Autodesk Inventor part; units mm, degrees
ref_plane "Work Plane1" through (29, -114.6, 0) normal (0, -1, 0) x (1, 0, 0)
ref_plane "YZ Plane" through (0, 0, 0) normal (1, 0, 0) x (0, 1, 0)
ref_plane "XZ Plane" through (0, 0, 0) normal (0, 1, 0) x (-1, 0, 0)
sketch "Sketch1" plane through (0, 0, 0) normal (0, 0, 1) x (1, 0, 0)
  line L0 (29, -258.2) -> (29, -233.2)
  line L1 (29, -233.2) -> (25, -233.2)
  line L2 (25, -233.2) -> (25, -193.2)
  line L3 (25, -193.2) -> (29, -193.2)
  line L4 (29, -193.2) -> (29, -168.2)
  line L5 (29, -168.2) -> (25, -168.2)
  line L6 (25, -168.2) -> (25, -128.2)
  line L7 (25, -128.2) -> (29, -128.2)
  line L8 (29, -128.2) -> (29, -103.2)
  line L9 (29, -103.2) -> (25, -103.2)
  line L10 (25, -103.2) -> (25, -63.2)
  line L11 (25, -63.2) -> (29, -63.2)
  line L12 (29, -63.2) -> (29, -36)
  line L13 (29, -36) -> (25, -36)
  line L14 (25, -36) -> (25, 4)
  line L15 (25, 4) -> (29, 4)
  line L16 (29, 4) -> (29, 29)
  line L17 (29, 29) -> (29, 25)
  line L18 (29, 25) -> (69, 25)
  line L19 (29, -258.2) -> (29, -254.2)
  line L20 (29, -254.2) -> (69, -254.2)
  line L21 (49, 25) -> (49, 50.1757)
  line L22 (69, -63.2) -> (69, -36)
  line L23 (73, -36) -> (73, 4)
  line L24 (69, -36) -> (73, -36)
  line L25 (73, 4) -> (69, 4)
  line L26 (73, -233.2) -> (73, -193.2)
  line L27 (73, -193.2) -> (69, -193.2)
  line L28 (69, -233.2) -> (73, -233.2)
  line L29 (69, -168.2) -> (73, -168.2)
  line L30 (73, -168.2) -> (73, -128.2)
  line L31 (73, -63.2) -> (69, -63.2)
  line L32 (69, -103.2) -> (73, -103.2)
  line L33 (73, -128.2) -> (69, -128.2)
  line L34 (73, -103.2) -> (73, -63.2)
  line L35 (69, 25) -> (69, 4)
  line L36 (69, -36) -> (69, -63.2)
  line L37 (69, -103.2) -> (69, -128.2)
  line L38 (69, -168.2) -> (69, -193.2)
  line L39 (69, -233.2) -> (69, -254.2)
  point P0 (0, 0)
  dimension "d1" = 40
  dimension "d2" = 4
  dimension "d3" = 40
  dimension "d4" = 40
  dimension "d5" = 40
  dimension "d6" = 40
  dimension "d7" = 279.2
extrude "Extrusion1" add sketch "Sketch1" along normal blind 4
sketch "Sketch2" plane through (0, 0, 4) normal (0, 0, 1) x (1, 0, 0)
  line L0 (25, -63.2) -> (25, -103.2)
  line L1 (25, -103.2) -> (29, -103.2)
  line L2 (29, -103.2) -> (29, -128.2)
  line L3 (29, -128.2) -> (25, -128.2)
  line L4 (25, -128.2) -> (25, -168.2)
  line L5 (25, -168.2) -> (29, -168.2)
  line L6 (29, -168.2) -> (29, -193.2)
  line L7 (29, -193.2) -> (25, -193.2)
  line L8 (25, -193.2) -> (25, -233.2)
  line L9 (25, -233.2) -> (29, -233.2)
  line L10 (29, -233.2) -> (29, -254.2)
  line L11 (29, -254.2) -> (69, -254.2)
  line L12 (69, -254.2) -> (69, -233.2)
  line L13 (69, -233.2) -> (73, -233.2)
  line L14 (73, -233.2) -> (73, -193.2)
  line L15 (73, -193.2) -> (69, -193.2)
  line L16 (69, -193.2) -> (69, -168.2)
  line L17 (69, -168.2) -> (73, -168.2)
  line L18 (73, -168.2) -> (73, -128.2)
  line L19 (73, -128.2) -> (69, -128.2)
  line L20 (69, -128.2) -> (69, -103.2)
  line L21 (69, -103.2) -> (73, -103.2)
  line L22 (73, -103.2) -> (73, -63.2)
  line L23 (73, -63.2) -> (69, -63.2)
  line L24 (69, -63.2) -> (69, -36)
  line L25 (69, -36) -> (73, -36)
  line L26 (73, -36) -> (73, 4)
  line L27 (73, 4) -> (69, 4)
  line L28 (69, 4) -> (69, 25)
  line L29 (69, 25) -> (29, 25)
  line L30 (29, 25) -> (29, 4)
  line L31 (29, 4) -> (25, 4)
  line L32 (25, 4) -> (25, -36)
  line L33 (25, -36) -> (29, -36)
  line L34 (29, -36) -> (29, -63.2)
  line L35 (29, -63.2) -> (25, -63.2)
  line L36 (44, 25) -> (54, 25)
  line L37 (54, 25) -> (54, 29)
  line L38 (54, 29) -> (44, 29)
  line L39 (44, 29) -> (44, 25)
  point P0 (0, 0)
  point P1 (49, 25)
  dimension "d10" = 10
  dimension "d11" = 4
extrude "Extrusion2" add sketch "Sketch2" against normal blind 4 contours L39 L38 L37 L29
ref_plane "Work Plane1" through (29, -114.6, 0) normal (0, -1, 0) x (1, 0, 0)
mirror "Mirror1" about plane through (29, -114.6, 0) normal (0, -1, 0) of "Extrusion2"
equation "\"d3\" = D"
equation "\"d4\" = D"
equation "\"d5\" = D"
equation "\"d6\" = D"
equation "\"d10\" = B"
equation "\"D\" = 40"
equation "\"B\" = 10"
properties part number "F3"
Read the model definition and answer for the solid it produces. Units are mm, in the model's axes. Coordinates: 2 decimals unless noted, no trailing zeros. Write each loop counter-clockwise with the first axis right and the second up, starting at its lowest first coordinate (ties: lowest second). Pieces come first, ordered by that corner, then holes. Notation, with made-up numbers: (46.25, -33) -> (54.25, -33) arc R20 ccw to (54.25, -11) -> close; hole circle Ø1 at (-8, -8). An arc over 180 degrees is marked (long way). Answer as a JSON object with one key per item and string values.
Q1. The part is cut by section B-B on x = 64. Give the vertices of the cut face in (y, z).
The answers:
{"outline": "(-254.2, 0) -> (25, 0) -> (25, 4) -> (-254.2, 4) -> close"}
Q2. The part is cut by section A-A on y = -182. Give the vertices of the cut face in (x, z), then the cut area to 3 significant figures.
The answers:
{"outline": "(29, 0) -> (69, 0) -> (69, 4) -> (29, 4) -> close", "area": "160 mm2"}
Q3. Consider line 1 (Y direction, x = 70, z = 2.45); line 2 (X direction, y = -55.5, z = 3.65); line 3 (Y direction, x = 43, z = 3.75). Determine where each line is inside the solid, lowest interval first. Write a range as [from, to].
The answers:
{"line 1": "y = [-233.2, -193.2], [-168.2, -128.2], [-103.2, -63.2], [-36, 4]", "line 2": "x = [29, 69]", "line 3": "y = [-254.2, 25]"}
Q4. Flat-ended cylindrical pins translate along their axes: pin 1 Ø1.2 at (y, z) = (-255.5, 2.5) entering from +X; pin 2 Ø1.5 at (y, z) = (-174, 1) entering from +X; pin 3 Ø1.2 at (x, z) = (28, 2) entering from +Y. Find the tip coordinate at first contact, or state that the pin passes through.
The answers:
{"pin 1": "stops at x = 54", "pin 2": "stops at x = 69", "pin 3": "stops at y = 4"}
